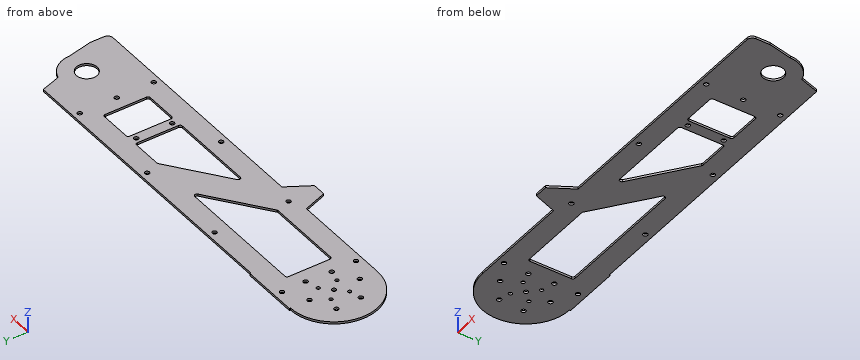
from build123d import *

# Parameters (mm, degrees)
SKETCH_1_R          = 2.1
SKETCH_1_R_2        = 2
SKETCH_1_R_3        = 9.52
SKETCH_1_R_4        = 2.05
SKETCH_1_R_5        = 1.65
EXTRUDE_1_DEPTH     = 2
SKETCH_3_W          = 52.726125437
SKETCH_3_H          = 0.98
EXTRUDE_2_DEPTH     = 2
SKETCH_2_R          = 2.05
SKETCH_2_W          = 32.809844138
SKETCH_2_H          = 42
CUT_EXTRUDE_1_DEPTH = 4
FILLET_1_R          = 2
FILLET_2_R          = 5


with BuildPart() as part:
    # 草图1 → 凸台-拉伸1 (new body)
    with BuildSketch(Plane.XY):
        with BuildLine():
            Line((-1.457142857, 39.854285714), (328.542857143, 39.854285714))
            Line((328.542857143, 39.854285714), (334.49569518, 22.070579719))
            ThreePointArc((334.49569518, 22.070579719), (346.78998397, 13.855798581), (351.542857143, -0.145714286))
            Line((351.542857143, -0.145714286), (356.542857143, -22.235997541))
            Line((356.542857143, -22.235997541), (356.542857143, -40.145714286))
            Line((356.542857143, -40.145714286), (328.542857143, -40.145714286))
            Line((328.542857143, -40.145714286), (126.194823947, -40.145714286))
            Line((126.194823947, -40.145714286), (113.608549915, -61.445714286))
            Line((113.608549915, -61.445714286), (101.341389716, -61.445714286))
            Line((101.341389716, -61.445714286), (93.462833584, -40.145714286))
            Line((93.462833584, -40.145714286), (-1.457142857, -40.145714286))
            ThreePointArc((-1.457142857, -40.145714286), (-41.457142857, -0.145714286), (-1.457142857, 39.854285714))
        make_face()
        with Locations((-1.457142857, -23.895714286)):
            Circle(SKETCH_1_R, mode=Mode.SUBTRACT)
        with Locations((18.028428728, -11.395714286)):
            Circle(SKETCH_1_R, mode=Mode.SUBTRACT)
        with Locations((-1.457142857, -0.145714286)):
            Circle(SKETCH_1_R_2, mode=Mode.SUBTRACT)
        with Locations((328.542857143, -0.145714286)):
            Circle(SKETCH_1_R_3, mode=Mode.SUBTRACT)
        with Locations((288.542857143, -0.145714286)):
            Circle(SKETCH_1_R_4, mode=Mode.SUBTRACT)
        with Locations((238.542857143, 16.354285714)):
            Circle(SKETCH_1_R_4, mode=Mode.SUBTRACT)
        with Locations(Location((238.542857143, -16.645714286, 0), (0, 0, 180))):
            Circle(SKETCH_1_R_4, mode=Mode.SUBTRACT)
        with Locations((-20.942714442, -11.395714286)):
            Circle(SKETCH_1_R, mode=Mode.SUBTRACT)
        with Locations((-22.025246197, 11.729285714)):
            Circle(SKETCH_1_R, mode=Mode.SUBTRACT)
        with Locations((-1.457142857, 22.354285714)):
            Circle(SKETCH_1_R, mode=Mode.SUBTRACT)
        with Locations((19.110960483, 11.729285714)):
            Circle(SKETCH_1_R, mode=Mode.SUBTRACT)
        with Locations((7.042857143, -8.645714286)):
            Circle(SKETCH_1_R_5, mode=Mode.SUBTRACT)
        with Locations((-9.957142857, -8.645714286)):
            Circle(SKETCH_1_R_5, mode=Mode.SUBTRACT)
        with Locations((-9.957142857, 8.354285714)):
            Circle(SKETCH_1_R_5, mode=Mode.SUBTRACT)
        with Locations((7.042857143, 8.354285714)):
            Circle(SKETCH_1_R_5, mode=Mode.SUBTRACT)
    extrude(amount=EXTRUDE_1_DEPTH)

    # 草图3 → 凸台-拉伸2 (add)
    with BuildSketch(Plane.XY.offset(2)):
        with Locations((24.905919862, 40.344285714)):
            Rectangle(SKETCH_3_W, SKETCH_3_H)
    extrude(amount=-EXTRUDE_2_DEPTH)

    # 草图2 → 切除-拉伸1 (cut)
    with BuildSketch(Plane.XY.offset(2)):
        with Locations((18.542857143, 33.854285714)):
            Circle(SKETCH_2_R)
        with Locations((108.542857143, 33.854285714)):
            Circle(SKETCH_2_R)
        with Locations((198.542857143, 33.854285714)):
            Circle(SKETCH_2_R)
        with Locations((288.542857143, 33.854285714)):
            Circle(SKETCH_2_R)
        with Locations((108.542857143, -34.145714286)):
            Circle(SKETCH_2_R)
        with Locations((198.542857143, -34.145714286)):
            Circle(SKETCH_2_R)
        with Locations((288.542857143, -34.145714286)):
            Circle(SKETCH_2_R)
        with Locations((18.542857143, -34.145714286)):
            Circle(SKETCH_2_R)
        Polygon((31.542857143, -21.145714286), (104.183898028, -21.145714286), (159.772133322, 20.854285714), (31.542857143, 20.854285714), align=None)
        Polygon((148.123425102, -21.145714286), (203.711660396, 20.854285714), (233.542857143, 20.854285714), (233.542857143, -21.145714286), align=None)
        with Locations((259.947779212, -0.145714286)):
            Rectangle(SKETCH_2_W, SKETCH_2_H)
    extrude(amount=-CUT_EXTRUDE_1_DEPTH, mode=Mode.SUBTRACT)

    # 圆角1
    fillet_1_edges = [part.edges().sort_by_distance(p)[0] for p in [
        (31.542857143, -21.145714286, 1),
        (31.542857143, 20.854285714, 1),
        (159.772133322, 20.854285714, 1),
        (104.183898028, -21.145714286, 1),
        (243.542857143, 20.854285714, 1),
        (276.352701281, 20.854285714, 1),
        (276.352701281, -21.145714286, 1),
        (243.542857143, -21.145714286, 1),
        (203.711660396, 20.854285714, 1),
        (233.542857143, 20.854285714, 1),
        (233.542857143, -21.145714286, 1),
        (148.123425102, -21.145714286, 1),
    ]]
    fillet(fillet_1_edges, radius=FILLET_1_R)

    # 圆角2
    fillet_2_edges = [part.edges().sort_by_distance(p)[0] for p in [
        (356.542857143, -40.145714286, 1),
    ]]
    fillet(fillet_2_edges, radius=FILLET_2_R)


solid = part.part
CAD build for the part. Positions are in the model's coordinates, mm. Give positions to 0.01 mm unless a question says otherwise; leave off trailing zeros. Write each loop counter-clockwise with the first axis right and the second up, starting at its lowest first coordinate (ties: lowest second). Pieces come first, ordered by that corner, then holes. Notation, with made-up numbers: M -36.5,33.5 L -12.5,33.5 A19 cw -12.5,54.5 Z; hole C 84,-19.75 d2. An arc over 180 degrees is marked long. Put each result on its own line as item: value. Start each with the question number.
(1) Band-saw the part on C-C, the plane y = -47. Write the cut outline in (x, z), and give its area (3 significant figures).
(2) Band-saw the part on D-D, the plane z = 1.4. Give the number of separate pieces and of enclosed holes in the cut face, and give its area (3 significant figures).
(3) Band-saw the part on A-A, the plane x = 254. Write the cut outline in (y, z).
(4) Probe L1, parallel to Y at x = 238, z = 1.6; L2, parallel to Y at x = 251, z = 1.05; L3, parallel to Y at x = 153, z = 1.75. List the from-to ranges inside material, lowest first.
(5) Band-saw the part on B-B, the plane x = 139. Write the cut outline in (y, z), and give its area (3 significant figures).
(6) Flat gauge pin, fed straight in: pin 1 Ø3.5 at (x, y) = (238.54, -16.65) entering from -Z. Where does the tip first touch, or does it go through?
Response values:
1. outline: M 96,0 L 122.14,0 L 122.14,2 L 96,2 Z
1. area: 52.3 mm2
2. separate pieces: 1
2. enclosed holes: 26
2. area: 22,400 mm2
3. outline: M -40.15,0 L -21.15,0 L -21.15,2 L -40.15,2 Z; M 20.85,0 L 39.85,0 L 39.85,2 L 20.85,2 Z
4. L1: y = -40.15 to -18.62, -14.67 to 14.38, 18.33 to 39.85
4. L2: y = -40.15 to -21.15, 20.85 to 39.85
4. L3: y = -40.15 to -20.82, -17.46 to 15.74, 20.85 to 39.85
5. outline: M -40.15,0 L 5.16,0 L 5.16,2 L -40.15,2 Z; M 20.85,0 L 39.85,0 L 39.85,2 L 20.85,2 Z
5. area: 129 mm2
6. pin 1: passes through
